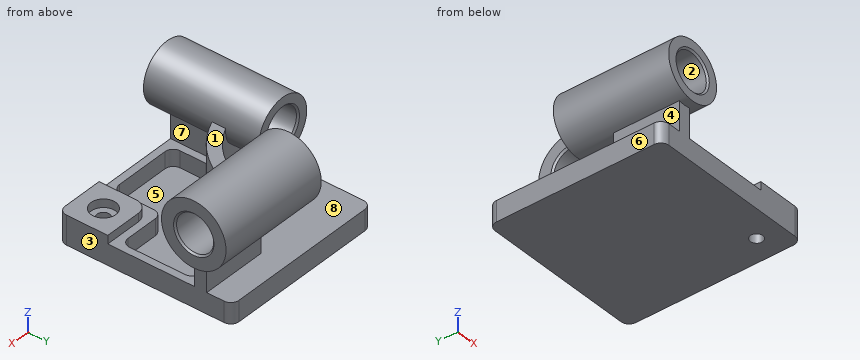
```python
from build123d import *

# Parameters (mm, degrees)
SKETCH1_W               = 205
SKETCH1_H               = 211
BOSS_EXTRUDE1_DEPTH     = 25
BOSS_EXTRUDE2_START     = -25
SKETCH2_W               = 60
SKETCH2_H               = 60
BOSS_EXTRUDE2_DEPTH     = 10
FILLET1_R               = 10
BOSS_EXTRUDE3_DEPTH     = 95
BOSS_EXTRUDE4_START     = 10
SKETCH5_R               = 35.166666667
BOSS_EXTRUDE4_DEPTH     = 140
SKETCH6_R               = 22.5
CUT_EXTRUDE1_DEPTH      = 140
BOSS_EXTRUDE5_START     = 10
SKETCH7_R               = 39.165
BOSS_EXTRUDE5_DEPTH     = 140
SKETCH8_R               = 22.5
CUT_EXTRUDE2_DEPTH      = 319.557726497
CUT_EXTRUDE5_DEPTH      = 35
CUT_EXTRUDE5_DEPTH_BACK = 15
CUT_EXTRUDE5_START      = -5
FILLET2_R               = 15
FILLET3_R               = 10
CHAMFER1_SIZE           = 2
CHAMFER2_SIZE           = 2


with BuildPart() as part:
    # Sketch1 → Boss-Extrude1 (new body)
    with BuildSketch(Plane.XY):
        with Locations((77.5, -74.5)):
            Rectangle(SKETCH1_W, SKETCH1_H)
    extrude(amount=BOSS_EXTRUDE1_DEPTH)

    # Sketch2 → Boss-Extrude2 (add)
    with BuildSketch(Plane(origin=(0, 0, 0), x_dir=(-1, 0, 0), z_dir=(0, 0, -1)).offset(BOSS_EXTRUDE2_START)):
        with Locations((-150, -150)):
            Rectangle(SKETCH2_W, SKETCH2_H)
    extrude(amount=-BOSS_EXTRUDE2_DEPTH)

    # Fillet1
    fillet1_edges = [part.edges().sort_by_distance(p)[0] for p in [
        (-25, 31, 12.5),
        (180, 31, 12.5),
        (180, -180, 17.5),
        (-25, -180, 12.5),
    ]]
    fillet(fillet1_edges, radius=FILLET1_R)

    # Sketch4 → Boss-Extrude3 (add)
    with BuildSketch(Plane.XY):
        with BuildLine():
            Line((0, -180), (0, -100))
            ThreePointArc((0, -100), (70.710678119, -70.710678119), (100, 0))
            Line((100, 0), (180, 0))
            Line((180, 0), (180, -15))
            Line((180, -15), (114.01754251, -15))
            ThreePointArc((114.01754251, -15), (81.317279836, -81.317279836), (15, -114.01754251))
            Line((15, -114.01754251), (15, -180))
            Line((15, -180), (0, -180))
        make_face()
    extrude(amount=BOSS_EXTRUDE3_DEPTH)

    # Sketch5 → Boss-Extrude4 (add)
    with BuildSketch(Plane.XZ.offset(180).offset(BOSS_EXTRUDE4_START)):
        with Locations((7.5, 95)):
            Circle(SKETCH5_R)
    extrude(amount=-BOSS_EXTRUDE4_DEPTH)

    # Sketch6 → Cut-Extrude1 (cut)
    with BuildSketch(Plane.XZ.offset(190)):
        with Locations((7.5, 95)):
            Circle(SKETCH6_R)
    extrude(amount=-CUT_EXTRUDE1_DEPTH, mode=Mode.SUBTRACT)

    # Sketch7 → Boss-Extrude5 (add)
    with BuildSketch(Plane(origin=(180, 0, 0), x_dir=(0, 0, -1), z_dir=(1, 0, 0)).offset(BOSS_EXTRUDE5_START)):
        with Locations(Location((-95, -7.5, 0), (0, 0, 90))):
            Circle(SKETCH7_R)
    extrude(amount=-BOSS_EXTRUDE5_DEPTH)

    # Sketch8 → Cut-Extrude2 (cut, through all)
    with BuildSketch(Plane(origin=(190, 0, 0), x_dir=(0, 0, -1), z_dir=(1, 0, 0))):
        with Locations(Location((-95, -7.5, 0), (0, 0, 90))):
            Circle(SKETCH8_R)
    extrude(amount=-CUT_EXTRUDE2_DEPTH, mode=Mode.SUBTRACT)

    # Sketch10 → Cut-Extrude5 (cut, two sides: drawn at the far end of the back side and taken through both)
    with BuildSketch(Plane.XY.offset(25).offset(CUT_EXTRUDE5_START - CUT_EXTRUDE5_DEPTH_BACK)):
        with BuildLine():
            Line((171, -33.428803755), (171, -101))
            ThreePointArc((171, -101), (168.071067812, -108.071067812), (161, -111))
            Line((161, -111), (121, -111))
            ThreePointArc((121, -111), (113.928932188, -113.928932188), (111, -121))
            Line((111, -121), (111, -161))
            ThreePointArc((111, -161), (108.071067812, -168.071067812), (101, -171))
            Line((101, -171), (34, -171))
            ThreePointArc((34, -171), (26.928932188, -168.071067812), (24, -161))
            Line((24, -161), (24, -136.527840403))
            Line((24, -136.527840403), (24, -121.655250606))
            ThreePointArc((24, -121.655250606), (87.681240867, -87.681240867), (121.655250606, -24))
            Line((121.655250606, -24), (132.503249765, -24))
            Line((132.503249765, -24), (164.331315018, -24))
            ThreePointArc((164.331315018, -24), (169.164347806, -27.654427173), (171, -33.428803755))
        make_face()
    extrude(amount=CUT_EXTRUDE5_DEPTH + CUT_EXTRUDE5_DEPTH_BACK, mode=Mode.SUBTRACT)

    # Sketch15 → CBORE for M8 Hex Head Bolt2 (revolve, cut)
    with BuildSketch(Plane(origin=(150, -150, 35), x_dir=(0, -1, 0), z_dir=(1, 0, 0))):
        Polygon((0, 0), (0, 35), (7.5, 35), (7.5, 10), (15, 10), (15, 0.025), (15.025, 0), align=None)
    revolve(axis=Axis((150, -150, 41.35), (0, 0, -1)), mode=Mode.SUBTRACT)

    # Fillet2
    fillet2_edges = [part.edges().sort_by_distance(p)[0] for p in [
        (120, -120, 30),
    ]]
    fillet(fillet2_edges, radius=FILLET2_R)

    # Fillet3
    fillet3_edges = [part.edges().sort_by_distance(p)[0] for p in [
        (24, -121.655250606, 15),
        (121.655250606, -24, 15),
    ]]
    fillet(fillet3_edges, radius=FILLET3_R)

    # Chamfer1
    chamfer1_edges = [part.edges().sort_by_distance(p)[0] for p in [
        (-15, -50, 95),
        (-15, -190, 95),
    ]]
    chamfer(chamfer1_edges, length=CHAMFER1_SIZE)

    # Chamfer2
    chamfer2_edges = [part.edges().sort_by_distance(p)[0] for p in [
        (50, -30, 95),
        (190, -30, 95),
    ]]
    chamfer(chamfer2_edges, length=CHAMFER2_SIZE)


solid = part.part
```
Model file for the job. Use its own axes, mm. Face numbers are marked on the shaded views. A direction names the side the tool comes from. Round coordinates to 2 decimals unless told otherwise and drop trailing zeros. Order: outer loops, then holes, each group sorted by start corner. A loop starts at its lowest first (then second) coordinate and runs counter-clockwise, first axis right, second up. Notation, with made-up numbers: M -32.5,-21 L -27.5,-21 A12 cw -27.5,-5 Z; hole C 75,26 d10. An arc over 180 degrees is marked long. Use CSV: the item, a comma, the result in double quotes.
Item 1: Saw through at C-C (y = -7.5). List the corners of the cut face in (x, z) (3 decimals), plus the area to 3 significant figures.
Worked answers:
outline,"M -25,0 L 180,0 L 180,55.835 L 190,55.835 L 190,70.5 L 188,72.5 L 52,72.5 L 50,70.5 L 50,55.835 L 99.718,55.835 L 99.718,25 L -25,25 Z; M 50,119.5 L 52,117.5 L 188,117.5 L 190,119.5 L 190,134.165 L 50,134.165 Z"
area,"12,300 mm²"
Item 2: Saw through at A-A (x = 150). List the corners of the cut face in (y, z) (3 decimals), plus the area to 3 significant figures.
Worked answers:
outline,"M -180,0 L -157.5,0 L -157.5,25 L -165,25 L -165,34.975 L -165.025,35 L -180,35 Z; M -142.5,0 L 31,0 L 31,25 L 0,25 L 0,56.56 A39.165 ccw long -15,56.56 L -15,25 L -24,25 L -24,5 L -111,5 L -111,25 L -120,25 L -120,35 L -134.975,35 L -135,34.975 L -135,25 L -142.5,25 Z; hole C -7.5,95 d45"
area,"7,150 mm²"
Item 3: Saw through at B-B (z = 123). List the corners of the cut face in (x, y), plus the area to 3 significant figures.
Worked answers:
outline,"M -13.78,-190 L 28.78,-190 L 28.78,-50 L -13.78,-50 Z; M 50,-34.88 L 190,-34.88 L 190,19.88 L 50,19.88 Z"
area,"13,600 mm²"
Item 4: Saw through at D-D (z = 15). List the corners of the cut face in (x, y).
Worked answers:
outline,"M -25,-170 A10 ccw -15,-180 L 170,-180 A10 ccw 180,-170 L 180,21 A10 ccw 170,31 L -15,31 A10 ccw -25,21 Z; hole M 24,-161 A10 ccw 34,-171 L 101,-171 A10 ccw 111,-161 L 111,-121 A10 cw 121,-111 L 161,-111 A10 ccw 171,-101 L 171,-33.43 A10 ccw 164.33,-24 L 129.61,-24 A10 ccw 119.94,-31.46 A124 cw 31.46,-119.94 A10 ccw 24,-129.61 Z; hole C 150,-150 d15"
Item 5: Which spindle directions (+Z, -Z, +X, -X, +Y, -Y) get a long thin tool onto all of the face, cutting with end or side? Do the marked faces 4, 5, 6, 7 and 8. Say none if no direction does.
Worked answers:
face 4,"-X, +Y, -Y"
face 5,"none"
face 6,"-Z, -X, +Y, -Y"
face 7,"-Y"
face 8,"-X, +Y"
Item 6: Pull direction X, two halves, no side cores. Call the marked faces 1, 2 and 3: released by +X, released by -X, zero draft, split by the parting line, or undercut.
Worked answers:
face 1,"zero draft"
face 2,"undercut"
face 3,"released by +X"
Item 7: Probe probe 1 along Y at (x, z) = (150, 31); probe 2 along X at (y, z) = (-150, 28); probe 3 along Z at (x, y) = (24, -77). List the from-to ranges inside material, lowest first.
Worked answers:
probe 1,"-180 to -165, -135 to -120, -15 to 0"
probe 2,"0 to 15, 120 to 135, 165 to 180"
probe 3,"0 to 25, 63.94 to 79.7, 110.3 to 126.06"
Item 8: Pin check, flat tips, straight feed: pin 1 (20 mm diameter, centred on y = -121.5, z = 12, fed in from -X); pin 2 (3 mm diameter, centred on x = 88, y = -142.5, fed in from -Z); pin 3 (10 mm diameter, centred on x = 144.5, z = 16, fed in from +Y); pin 4 (16 mm diameter, centred on y = -142, z = 15.5, fed in from +X). Stop position of each tip, or through.
Worked answers:
pin 1,"x = -25"
pin 2,"z = 0"
pin 3,"y = 31"
pin 4,"x = 180"
